Build history of the part. All positions in model axes, mm. Face numbers are marked on the shaded views. A direction names the side the tool comes from. Coordinates: 2 decimals unless noted, no trailing zeros. Write each loop counter-clockwise with the first axis right and the second up, starting at its lowest first coordinate (ties: lowest second). Pieces come first, ordered by that corner, then holes.
```python
from build123d import *

# Parameters (mm, degrees)
F1_DEPTH = 12.7
F2_DEPTH = 12.7


with BuildPart() as f1:
    # F0 (on Front) → F1 (new body, symmetric)
    with BuildSketch(Plane.XZ):
        Polygon((28.504521, 70.64042), (28.504521, -42.545328), (38.498788, -56.35958), (41.204521, -56.35958), (41.204521, 70.64042), align=None)
    extrude(amount=F1_DEPTH, both=True)

    # F0 (on Front) → F2 (join, symmetric)
    with BuildSketch(Plane.XZ):
        Polygon((-53.38255, 70.64042), (-66.08255, 70.64042), (-66.08255, -56.35958), (-53.38255, -56.35958), (-53.38255, -0.88598), (-53.38255, 56.82433), (28.504521, -56.35958), (38.498788, -56.35958), (28.504521, -42.545328), align=None)
    extrude(amount=F2_DEPTH, both=True)


solid = f1.part
```
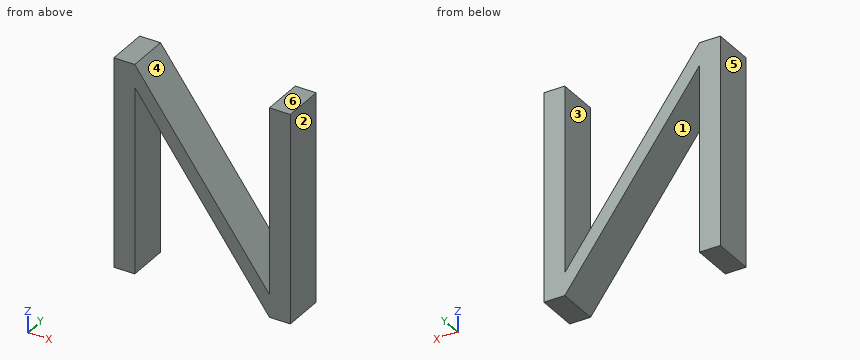
1. Saw through at B-B on y = -2.75. List the corners of the cut face in (x, z), plus the area to 3 significant figures.
Computed values:
outline: (-66.08, -56.36) - (-53.38, -56.36) - (-53.38, 56.82) - (28.5, -56.36) - (41.2, -56.36) - (41.2, 70.64) - (28.5, 70.64) - (28.5, -42.55) - (-53.38, 70.64) - (-66.08, 70.64) - close
area: 4,360 mm2
2. 3-axis set-ups, long thin cutter, end or side, ignore diameter. For the marked faces 1, 2 and 3: which of +Z, -Z, +X, -X, +Y, -Y reach the whole face in a straight line?
Computed values:
face 1: -Z, +Y, -Y
face 2: +Z, -Z, +X, +Y, -Y
face 3: +Z, +Y, -Y
3. Probe line 1 along X through (y, z) = (-2, -24); line 2 along X through (y, z) = (3, -33); line 3 along X through (y, z) = (8.5, 57.5). List the from-to ranges inside material, lowest first.
Computed values:
line 1: x = -66.08 to -53.38, 5.09 to 15.09, 28.5 to 41.2
line 2: x = -66.08 to -53.38, 11.6 to 21.6, 28.5 to 41.2
line 3: x = -66.08 to -43.88, 28.5 to 41.2
4. Saw through at A-A on z = 63.5. List the corners of the cut face in (x, y), plus the area to 3 significant figures.
Computed values:
outline: (-66.08, -12.7) - (-48.22, -12.7) - (-48.22, 12.7) - (-66.08, 12.7) - close; (28.5, -12.7) - (41.2, -12.7) - (41.2, 12.7) - (28.5, 12.7) - close
area: 776 mm2
5. Saw through at D-D on x = -14. List the corners of the cut face in (y, z).
Computed values:
outline: (-12.7, 2.39) - (12.7, 2.39) - (12.7, 16.21) - (-12.7, 16.21) - close
6. Flat gauge pins, fed straight in: pin 1 (4 mm diameter, centred on x = -49, y = -4.5, fed in from +Z); pin 2 (3 mm diameter, centred on x = 13.5, y = 6.5, fed in from +Z); pin 3 (8 mm diameter, centred on x = 6.5, y = 1, fed in from -Z). Where does each tip first touch, or does it go through?
Computed values:
pin 1: stops at z = 67.35
pin 2: stops at z = -19.73
pin 3: stops at z = -31.47
7. Mould opens along X. For the marked faces 4, 5 and 6 say: +X half, -X half, draft (parallel to the pull), parting line (faces both ways), or undercut.
Computed values:
face 4: undercut
face 5: -X half
face 6: draft
8. Saw through at C-C on z = -5.5. List the corners of the cut face in (x, y).
Computed values:
outline: (-66.08, -12.7) - (-53.38, -12.7) - (-53.38, 12.7) - (-66.08, 12.7) - close; (-8.29, -12.7) - (1.7, -12.7) - (1.7, 12.7) - (-8.29, 12.7) - close; (28.5, -12.7) - (41.2, -12.7) - (41.2, 12.7) - (28.5, 12.7) - close
